For this review, use the dimensioned drawing (mm, ordinates from the lowest corner) and the shaded views. A direction names the side the tool comes from. Round coordinates to 2 decimals unless told otherwise and drop trailing zeros. Write each loop counter-clockwise with the first axis right and the second up, starting at its lowest first coordinate (ties: lowest second). Pieces come first, ordered by that corner, then holes. Notation, with made-up numbers: (71.5, -8.5) - (101.5, -8.5) arc R27 cw to (101.5, 16.5) - close; hole circle Ø5 at (70.25, -23.75). An arc over 180 degrees is marked (long way). Return JSON: item names as keys, results as strings.
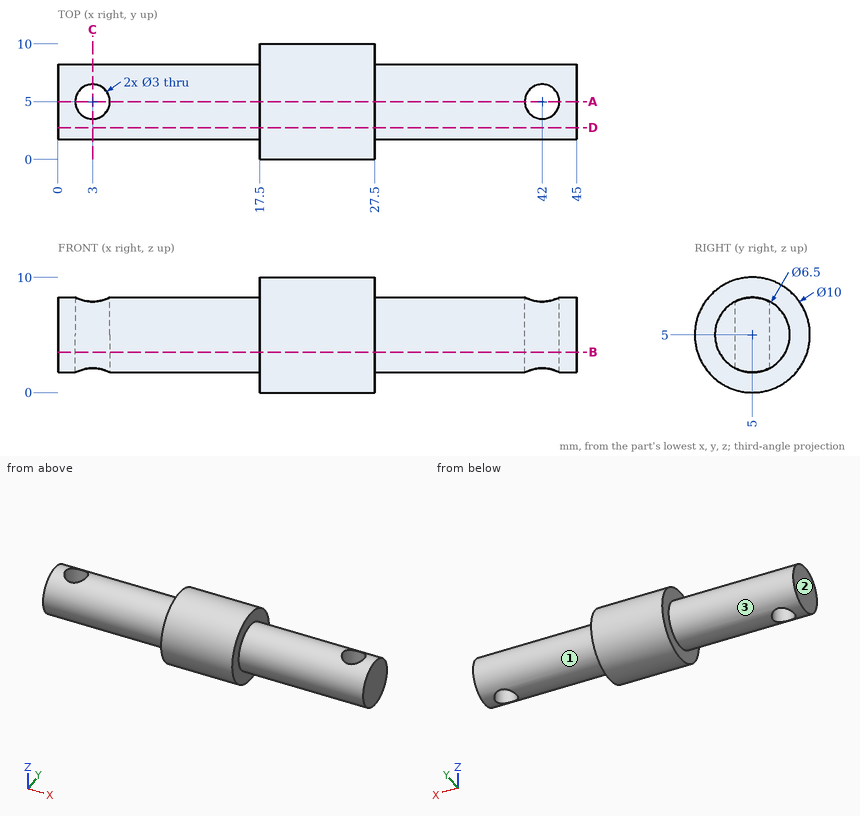
(1) Clearance check with flat-ended pins moving along their axes: pin 1 Ø1.5 at (y, z) = (8.5, 3) entering from -X; pin 2 Ø3.5 at (x, y) = (3, 5) entering from -Z; pin 3 Ø2 at (y, z) = (6.5, 1.5) entering from +X; pin 4 Ø1.5 at (x, z) = (24, 3) entering from -Y. State where each tip first meets the part, or that it passes through.
Filled in:
{"pin 1": "stops at x = 17.5", "pin 2": "stops at z = 1.75", "pin 3": "stops at x = 45", "pin 4": "stops at y = 0.16"}
(2) Add section C-C (x = 3). Write out the cut boundary in (y, z), plus the area to 3 significant figures.
Filled in:
{"outline": "(3.5, 2.12) - (3.5, 7.88) arc R3.25 ccw to start; (6.5, 2.12) arc R3.25 ccw to (6.5, 7.88) - close", "area": "14.4 mm2"}
(3) Add section A-A (y = 5). Write out the cut boundary in (x, z), plus the area to 4 significant figures.
Filled in:
{"outline": "(0, 1.75) - (1.5, 1.75) - (1.5, 8.25) - (0, 8.25) - close; (4.5, 1.75) - (17.5, 1.75) - (17.5, 0) - (27.5, 0) - (27.5, 1.75) - (40.5, 1.75) - (40.5, 8.25) - (27.5, 8.25) - (27.5, 10) - (17.5, 10) - (17.5, 8.25) - (4.5, 8.25) - close; (43.5, 1.75) - (45, 1.75) - (45, 8.25) - (43.5, 8.25) - close", "area": "288.5 mm2"}
(4) Add section B-B (z = 3.5). Write out the cut boundary in (x, y).
Filled in:
{"outline": "(0, 2.12) - (17.5, 2.12) - (17.5, 0.23) - (27.5, 0.23) - (27.5, 2.12) - (45, 2.12) - (45, 7.88) - (27.5, 7.88) - (27.5, 9.77) - (17.5, 9.77) - (17.5, 7.88) - (0, 7.88) - close; hole circle Ø3 at (3, 5); hole circle Ø3 at (42, 5)"}
(5) Add section D-D (y = 2.75). Write out the cut boundary in (x, z).
Filled in:
{"outline": "(0, 2.65) - (17.5, 2.65) - (17.5, 0.53) - (27.5, 0.53) - (27.5, 2.65) - (45, 2.65) - (45, 7.35) - (27.5, 7.35) - (27.5, 9.47) - (17.5, 9.47) - (17.5, 7.35) - (0, 7.35) - close"}
(6) Wall thickness on line 1 (X direction, y = 5, z = 3.15); line 2 (X direction, y = 2.25, z = 8.25); line 3 (X direction, y = 6.25, z = 7): over which ranges is each line inside the solid? List them lowest first.
Filled in:
{"line 1": "x = 0 to 1.5, 4.5 to 40.5, 43.5 to 45", "line 2": "x = 17.5 to 27.5", "line 3": "x = 0 to 2.17, 3.83 to 41.17, 42.83 to 45"}
(7) For the marked faces 1, 2 and 3, list the 3-axis set-ups (+Z, -Z, +X, -X, +Y, -Y) from which the entire face can be reached by the end or side of a thin tool; tool diameter is ignored.
Filled in:
{"face 1": "+X", "face 2": "+Z, -Z, -X, +Y, -Y", "face 3": "-X"}
